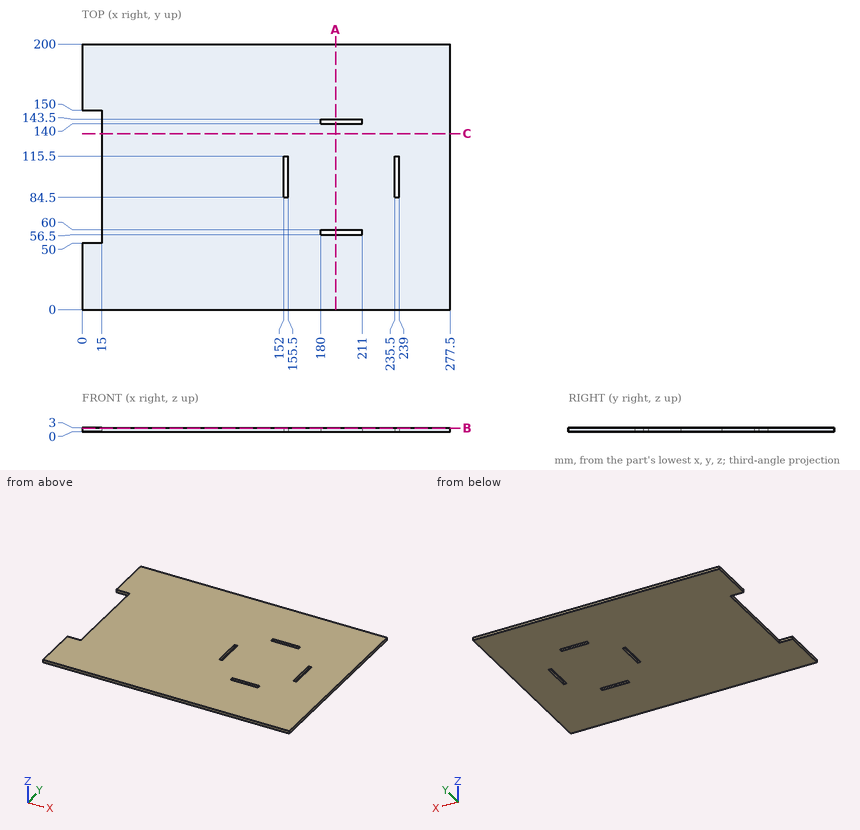
Design review of the part shown in the three views and the two pictorial views. Dimensions are in mm from the part's minimum x, y and z. Round coordinates to 2 decimals unless told otherwise and drop trailing zeros. Write each loop counter-clockwise with the first axis right and the second up, starting at its lowest first coordinate (ties: lowest second). Pieces come first, ordered by that corner, then holes. Notation, with made-up numbers: (51, 79.5) - (61, 79.5) arc R20 cw to (61, 87.5) - close; hole circle Ø5 at (78, 51.5). An arc over 180 degrees is marked (long way). Return JSON: item names as keys, results as strings. Group by question number.
Item 1: We need section A-A on x = 191. Write out the cut boundary in (y, z), and give its area (3 significant figures).
Item 2: Insertion check: P1, Ø0.9, axis at y = 58.5, z = 2, coming from the -X side. The pin has a flat end and moves straight along its axis. Give the tip position at first contact, or say it passes through.
Item 3: For probe 1 along X at (y, z) = (96, 1.3); probe 2 along X at (y, z) = (123.5, 2.8), list the stretches that pass through material, from the lowest coordinate up. Write a range as [from, to].
Item 4: We need section B-B on z = 2.5. Write out the cut boundary in (x, y).
Item 5: We need section C-C on y = 132.5. Write out the cut boundary in (x, z).
Model answer:
{
 "1": {"outline": "(0, 0) - (56.5, 0) - (56.5, 3) - (0, 3) - close; (60, 0) - (140, 0) - (140, 3) - (60, 3) - close; (143.5, 0) - (200, 0) - (200, 3) - (143.5, 3) - close", "area": "579 mm²"},
 "2": {"P1": "stops at x = 15"},
 "3": {"probe 1": "x = [15, 152], [155.5, 235.5], [239, 277.5]", "probe 2": "x = [15, 277.5]"},
 "4": {"outline": "(0, 0) - (277.5, 0) - (277.5, 200) - (0, 200) - (0, 150) - (15, 150) - (15, 50) - (0, 50) - close; hole (152, 84.5) - (155.5, 84.5) - (155.5, 115.5) - (152, 115.5) - close; hole (180, 56.5) - (211, 56.5) - (211, 60) - (180, 60) - close; hole (180, 140) - (211, 140) - (211, 143.5) - (180, 143.5) - close; hole (235.5, 84.5) - (239, 84.5) - (239, 115.5) - (235.5, 115.5) - close"},
 "5": {"outline": "(15, 0) - (277.5, 0) - (277.5, 3) - (15, 3) - close"}
}
